```python
from build123d import *

# Parameters (mm, degrees)
F0_R     = 26.8224
F0_R_2   = 11.049
F1_DEPTH = 6.985
F0_R_3   = 31.75
F2_DEPTH = 2.54
F3_R     = 26.8224
F3_R_2   = 11.049
F3_R_3   = 5.08
F4_DEPTH = 1.5875
F5_R     = 15.207522
F5_R_2   = 5.08
F6_DEPTH = 25.4


with BuildPart() as f1:
    # F0 (on Top) → F1 (new body)
    with BuildSketch(Plane.XY):
        Circle(F0_R)
        Circle(F0_R_2, mode=Mode.SUBTRACT)
    extrude(amount=F1_DEPTH)

    # F0 (on Top) → F2 (join)
    with BuildSketch(Plane.XY):
        Circle(F0_R_3)
        Circle(F0_R, mode=Mode.SUBTRACT)
    extrude(amount=F2_DEPTH)

    # F3 (on face) → F4 (join)
    with BuildSketch(Plane.XY.offset(6.985)):
        Circle(F3_R)
        Circle(F3_R_2, mode=Mode.SUBTRACT)
        Circle(F3_R_2)
        Circle(F3_R_3, mode=Mode.SUBTRACT)
    extrude(amount=F4_DEPTH)

    # F5 (on face) → F6 (join)
    with BuildSketch(Plane.XY.offset(8.5725)):
        Circle(F5_R)
        Circle(F5_R_2, mode=Mode.SUBTRACT)
    extrude(amount=F6_DEPTH)


solid = f1.part
```
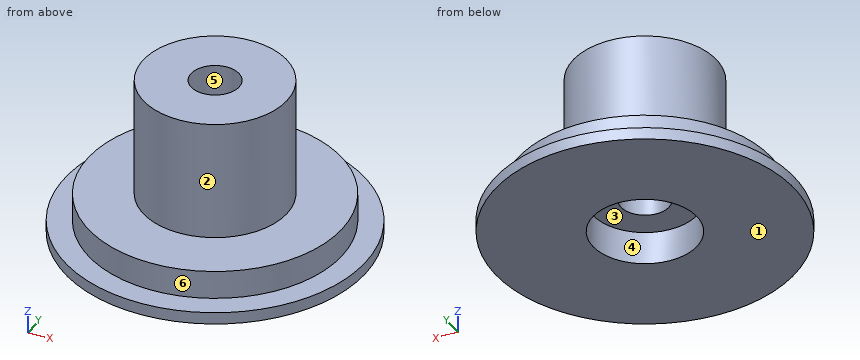
Can you work these out from the model? Positions are in its coordinate system, mm. Face numbers are marked on the shaded views. A direction names the side the tool comes from. Give positions to 0.01 mm unless a question says otherwise; leave off trailing zeros. Order: outer loops, then holes, each group sorted by start corner. A loop starts at its lowest first (then second) coordinate and runs counter-clockwise, first axis right, second up. Notation, with made-up numbers: (25, -27) - (84, -27) arc R33 ccw to (84, 2) - close; hole circle Ø5 at (-28.5, 13). An arc over 180 degrees is marked (long way). Use a Markdown table: item, result. Add a question column.
Q1. I'm going to push flat-ended pins straight in: pin 1 (12 mm diameter, centred on y = 0.5, z = 9.5, fed in from -X); pin 2 (5 mm diameter, centred on x = 6, z = 17.5, fed in from -Y); pin 3 (1 mm diameter, centred on y = 12.5, z = 19, fed in from +X). Where does each tip first touch, or does it pass through?
Q2. If we section it at C-C on z = 28: Write out the boundary of the cut face in (x, y), plus the area to 3 significant figures.
Q3. Please list where these lines run through material, in increasing order: line 1 along Y through (x, z) = (0, 13); line 2 along Z through (x, y) = (-16, 27); line 3 along Z through (x, y) = (3.5, -22).
Q4. If we section it at D-D on y = 16: Write out the boundary of the cut face in (x, z).
Q5. On a 3-axis mill with a long thin cutter (end or side, diameter ignored), from which of +Z, -Z, +X, -X, +Y, -Y can I reach the whole of each face in a straight line? I mean the marked faces 4, 5 and 6. Say none if no direction works.
Q6. If we mould it in two halves opening along Y, with no side actions, what happens to the marked faces 1, 2 and 3? For each: released by +Y, released by -Y, zero draft, split by the parting line, or undercut.
Answers follow:
| question | item | result |
|---|---|---|
| 1 | pin 1 | stops at x = -26.82 |
| 1 | pin 2 | stops at y = -14.8 |
| 1 | pin 3 | stops at x = 9.34 |
| 2 | outline | circle Ø30.42 at (0, 0); hole circle Ø10.16 at (0, 0) |
| 2 | area | 645 mm^2 |
| 3 | line 1 | y = -15.21 to -5.08, 5.08 to 15.21 |
| 3 | line 2 | z = 0 to 2.54 |
| 3 | line 3 | z = 0 to 8.57 |
| 4 | outline | (-27.42, 0) - (27.42, 0) - (27.42, 2.54) - (21.53, 2.54) - (21.53, 8.57) - (-21.53, 8.57) - (-21.53, 2.54) - (-27.42, 2.54) - close |
| 5 | face 4 | -Z |
| 5 | face 5 | +Z, -Z |
| 5 | face 6 | +Z |
| 6 | face 1 | zero draft |
| 6 | face 2 | split by the parting line |
| 6 | face 3 | undercut |
